Autodesk Inventor part; units mm, degrees
ref_plane "A_XY" through (2.5, 3, 0) normal (0, 0, 1) x (1, 0, 0)
ref_plane "A_YZ" through (2.5, 3, 0) normal (1, 0, 0) x (0, 1, 0)
ref_plane "A_ZX" through (2.5, 3, 0) normal (0, 1, 0) x (0, 0, 1)
sketch "Sketch_1" plane through (0, 0, 0) normal (0, 0, 1) x (1, 0, 0)
  arc A0 (3.6737, 5.7073) -> (2.9784, 1.0462) centre (2.5, 3.5) ccw
  line L0 (2.9784, 1.0462) -> (12.3318, 2.8697)
  arc A1 (13.6089, 2.6955) -> (12.3318, 2.8697) centre (12.7145, 0.9067) ccw
  line L1 (13.6089, 2.6955) -> (16.8654, 1.0673)
  arc A2 (16.8654, 1.0673) -> (17.6821, 1.1275) centre (17.2232, 1.7828) ccw
  line L2 (17.6821, 1.1275) -> (25, 6.2516)
  line L3 (25, 6.2516) -> (24.4264, 7.0707)
  line L4 (24.4264, 7.0707) -> (18.182, 2.6984)
  arc A3 (16.1405, 2.5478) -> (18.182, 2.6984) centre (17.0349, 4.3367) ccw
  line L5 (16.1405, 2.5478) -> (4.8361, 8.2)
  line L6 (4.8361, 8.2) -> (3.6737, 5.7073)
  circle A4 centre (8, 4) radius 0.75
extrude "Extrusion1" add sketch "Sketch_1" along normal mid plane 12
sketch "Sketch_2" plane through (0, 0, 0) normal (0, 0, 1) x (1, 0, 0)
  circle A0 centre (2.5, 3.5) radius 3.8829
extrude "Extrusion2" cut sketch "Sketch_2" along normal mid plane 10.5
sketch "Sketch_3" plane through (0, 0, 0) normal (0, 1, 0) x (-1, 0, 0)
  line L0 (-13, -5) -> (-15, -3)
  line L1 (-15, -3) -> (-22, -3)
  arc A0 (-22, 3) -> (-22, -3) centre (-22, 0) ccw
  line L2 (-22, 3) -> (-15, 3)
  line L3 (-15, 3) -> (-13, 5)
  line L4 (-13, 5) -> (-13, 6)
  line L5 (-13, 6) -> (-30, 6)
  line L6 (-30, 6) -> (-30, -6)
  line L7 (-30, -6) -> (-13, -6)
  line L8 (-13, -6) -> (-13, -5)
extrude "Extrusion3" cut sketch "Sketch_3" along normal blind 15
sketch "Sketch_4" plane through (2.5, 0, 0) normal (1, 0, 0) x (0, 0, -1)
  line L0 (6.75, 3) -> (-6.75, 3)
  arc A0 (-6.6154, 3.3413) -> (-6.75, 3) centre (-6.25, 3) ccw
  line L1 (-6.6154, 3.3413) -> (-6, 4)
  line L2 (-6, 4) -> (6, 4)
  line L3 (6, 4) -> (6.6154, 3.3413)
  arc A1 (6.75, 3) -> (6.6154, 3.3413) centre (6.25, 3) ccw
  line L4 (6.75, 3) -> (-6.75, 3)
revolve "Revolution1" add sketch "Sketch_4" angle 360 about axis through (2.5, 3, -6.75) along (0, 0, -1)
ref_plane "A_XY" through (2.5, 3, 0) normal (0, 0, 1) x (1, 0, 0)
ref_plane "A_YZ" through (2.5, 3, 0) normal (1, 0, 0) x (0, 1, 0)
ref_plane "A_ZX" through (2.5, 3, 0) normal (0, 1, 0) x (0, 0, 1)
ref_plane "B_XY" through (8, 4, 0) normal (0, 0, 1) x (1, 0, 0)
ref_plane "B_YZ" through (8, 4, 0) normal (1, 0, 0) x (0, 1, 0)
ref_plane "B_ZX" through (8, 4, 0) normal (0, 1, 0) x (0, 0, 1)
properties part number "PKWS1-HOOK"
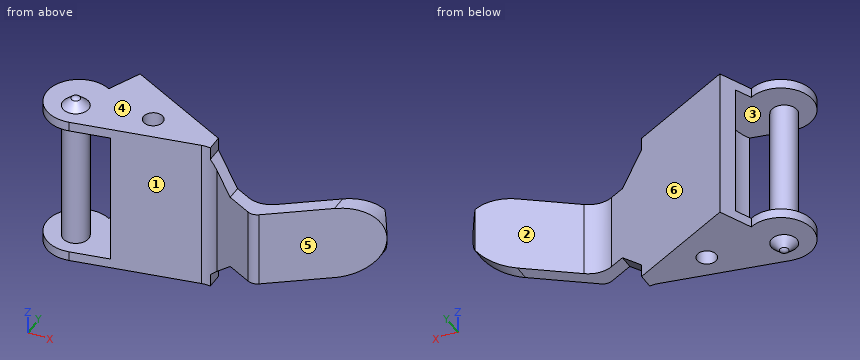
Can you work these out from the model? Positions are in its coordinate system, mm. Face numbers are marked on the shaded views. A direction names the side the tool comes from. Coordinates: 2 decimals unless noted, no trailing zeros. Loops run counter-clockwise (first coordinate to the right, second up) from the corner with the lowest first, then second, coordinate; pieces in that order, holes last. Notation, with made-up numbers: M 43.25,28 L 88.25,28 A35 cw 88.25,62 Z; hole C 5,-31 d6. An arc over 180 degrees is marked long. Put each result on its own line as item: value. Start each with the question number.
(1) Imagine slicing it at D-D on x = 8. List the corners of the cut face in (y, z) for me, and give its area (3 significant figures).
(2) Will these pins go through, and if not, where does the flat tip stop? pin 1 Ø3.5 at (x, y) = (17.5, 3) entering from -Z; pin 2 Ø2 at (y, z) = (4.5, -1) entering from -X; pin 3 Ø2 at (x, y) = (8, 4) entering from -Z.
(3) Imagine slicing it at B-B on y = 4.5. List the corners of the cut face in (x, z) for me (3 decimals).
(4) Imagine slicing it at A-A on z = -2.5. List the corners of the cut face in (x, y) for me, and give its area (3 significant figures).
(5) I need wall thicknesses on probe 1 along X at (y, z) = (3.75, 1.75); probe 2 along Y at (x, z) = (7.5, 5.5); probe 3 along Y at (x, z) = (8, -0.75). Which ranges of each line are inside material? Lowest first, please.
(6) We'd pull the mould along X, two halves only. Please class the marked faces 4, 5 and 6: +X half, -X half, draft (parallel to the pull), parting line (faces both ways), or undercut.
(7) Which directions (+Z, -Z, +X, -X, +Y, -Y) give clear straight access to the entire face, cutting with the end or side of a thin tool? Please do the marked faces 1, 2 and 3.
(8) Imagine slicing it at C-C on y = 6.5. List the corners of the cut face in (x, z) for me, and give its area (3 significant figures).
Worked answers:
1. outline: M 2.03,-6 L 3.25,-6 L 3.25,6 L 2.03,6 Z; M 4.75,-6 L 6.62,-6 L 6.62,6 L 4.75,6 Z
1. area: 37.1 mm2
2. pin 1: stops at z = -3
2. pin 2: stops at x = 1.63
2. pin 3: stops at z = -6
3. outline: M 0.209,-6 L 7.441,-6 L 7.441,6 L 0.209,6 L 0.209,5.25 L 6.252,5.25 L 6.252,-5.25 L 0.209,-5.25 Z; M 8.559,-6 L 12.236,-6 L 12.236,6 L 8.559,6 Z; M 20.755,-3 L 22,-3 A3 ccw 22.498,-2.958 L 22.498,2.958 A3 ccw 22,3 L 20.755,3 Z
4. outline: C 2.5,3 d2; M 4.26,6.96 A3.88 cw 5.89,1.61 L 12.33,2.87 A2 cw 13.61,2.7 L 16.87,1.07 A0.8 ccw 17.68,1.13 L 23.66,5.31 L 23.66,6.53 L 18.18,2.7 A2 cw 16.14,2.55 L 4.84,8.2 Z; hole C 8,4 d1.5
4. area: 40.9 mm2
5. probe 1: x = 1.84 to 3.16, 6.37 to 7.29, 8.71 to 13.74, 19.68 to 21.43
5. probe 2: y = 1.93 to 3.44, 4.56 to 6.87
5. probe 3: y = 2.03 to 3.25, 4.75 to 6.62
6. face 4: draft
6. face 5: +X half
6. face 6: undercut
7. face 1: +Z, -Z, -Y
7. face 2: +Z, -Z, +Y
7. face 3: none
8. outline: M 4.04,-6 L 8.24,-6 L 8.24,6 L 4.04,6 L 4.04,5.25 L 4.97,5.25 L 4.97,-5.25 L 4.04,-5.25 Z; M 23.61,-2.53 A3 ccw 24.83,-1.01 L 24.83,1.01 A3 ccw 23.61,2.53 Z
8. area: 45.4 mm2
